Part print with two shaded views. Sizes in mm from the minimum x, y, z corner. A direction names the side the tool comes from. Round coordinates to 2 decimals unless told otherwise and drop trailing zeros. Loops run counter-clockwise (first coordinate to the right, second up) from the corner with the lowest first, then second, coordinate; pieces in that order, holes last. Notation, with made-up numbers: (-9, -21.75) -> (14, -21.75) arc R13 cw to (14, -1.75) -> close; hole circle Ø10 at (80, -2.75). An arc over 180 degrees is marked (long way). Use a Markdown table: item, result. Add a question column.
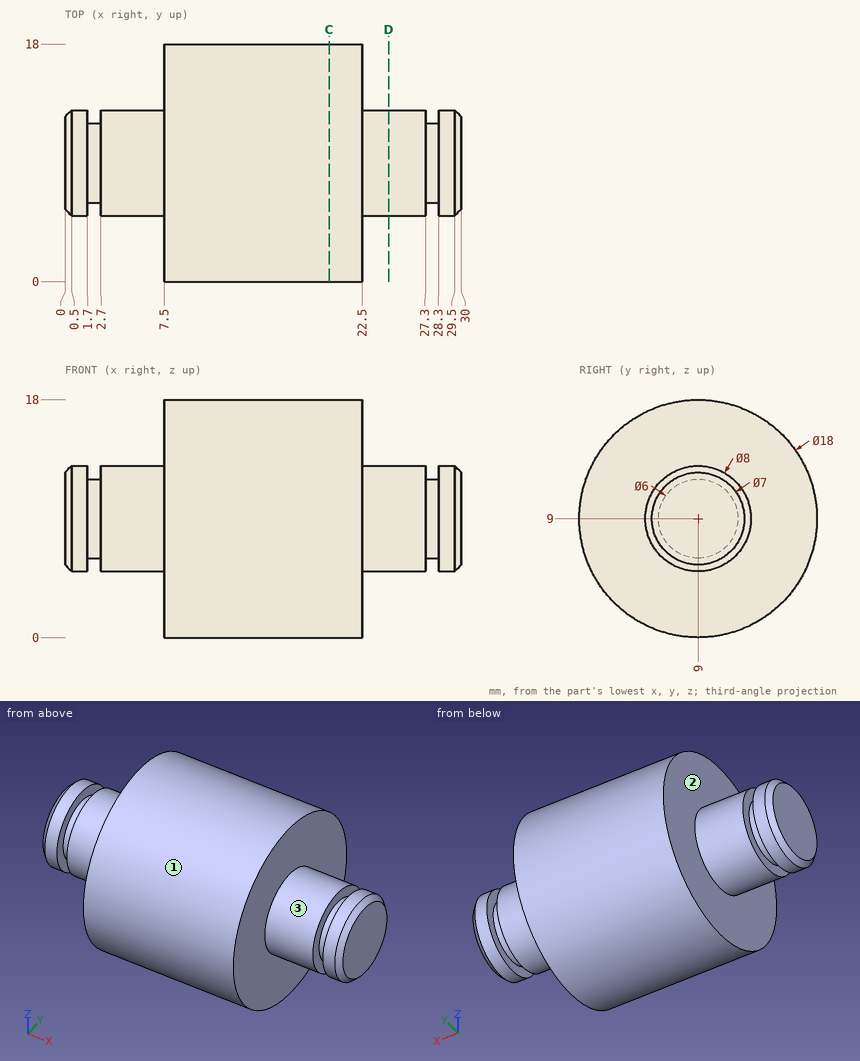
1) Cut at D-D on x = 24.5. Write the cut outline in (y, z), and give its area (3 significant figures).
2) Wall check: probe 1 along X at (y, z) = (5.5, 10.75); probe 2 along X at (y, z) = (14.25, 4.25); probe 3 along Z at (x, y) = (13.5, 3.5). Give the ranges that are in metal, low to high. Write a range as from..to.
3) Pin check, flat tips, straight feed: pin 1 Ø1.5 at (y, z) = (9, 3) entering from -X; pin 2 Ø5 at (x, z) = (7, 14) entering from +Y; pin 3 Ø2 at (x, z) = (12, 2) entering from +Y; pin 4 Ø1 at (x, y) = (4, 14) entering from -Z. Stop position of each tip, or through.
4) Cut at C-C on x = 20. Write the cut outline in (y, z).
5) Tool access for the marked faces 1, 2 and 3: list every direction of +Z, -Z, +X, -X, +Y, -Y with a clear straight run to the whole face (end or side of a thin tool).
Established:
| question | item | result |
|---|---|---|
| 1 | outline | circle Ø8 at (9, 9) |
| 1 | area | 50.3 mm^2 |
| 2 | probe 1 | x = 0.41..1.7, 2.7..27.3, 28.3..29.59 |
| 2 | probe 2 | x = 7.5..22.5 |
| 2 | probe 3 | z = 1.88..16.12 |
| 3 | pin 1 | stops at x = 7.5 |
| 3 | pin 2 | stops at y = 17.63 |
| 3 | pin 3 | stops at y = 15.71 |
| 3 | pin 4 | passes through |
| 4 | outline | circle Ø18 at (9, 9) |
| 5 | face 1 | +X, -X |
| 5 | face 2 | -X |
| 5 | face 3 | +X |
